```python
from build123d import *

# Parameters (mm, degrees)
F3_R        = 22.5
F4_DEPTH    = 80
F2_R        = 7.5
F0_R        = 17.5
F4_FACE_R   = 22.5
F4_FACE_R_2 = 7.5
F6_DEPTH    = 2


with BuildPart() as f4:
    # F3 (on Top) → F4 (new body)
    with BuildSketch(Plane.XY):
        Circle(F3_R)
    extrude(amount=F4_DEPTH)

    # F2 (on offset) → F5 section 0
    with BuildSketch(Plane.XY.offset(80)):
        Circle(F2_R)
    # F0 (on Top) → F5 section 1
    with BuildSketch(Plane.XY):
        Circle(F0_R)
    loft(mode=Mode.SUBTRACT)

    # F2 (on offset) + F4_face (on face) → F6 (join)
    with BuildSketch(Plane.XY.offset(80)):
        Circle(F2_R)
    with BuildSketch(Plane.XY.offset(80)):
        Circle(F4_FACE_R)
        Circle(F4_FACE_R_2, mode=Mode.SUBTRACT)
    extrude(amount=F6_DEPTH)


solid = f4.part
```
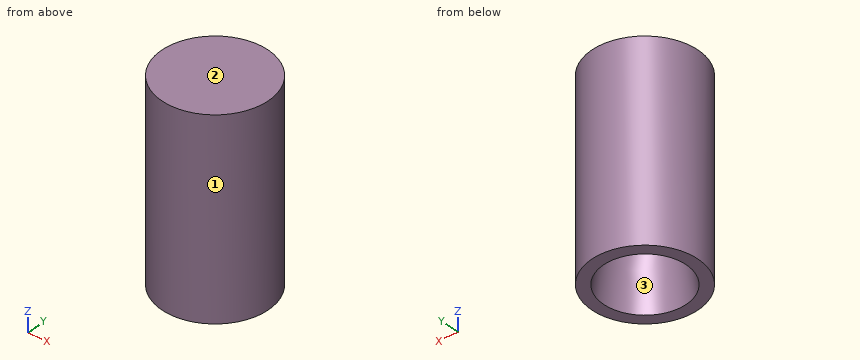
Model file for the job. Use its own axes, mm. Face numbers are marked on the shaded views. Give positions to 0.01 mm unless a question says otherwise; leave off trailing zeros. Order: outer loops, then holes, each group sorted by start corner. A loop starts at its lowest first (then second) coordinate and runs counter-clockwise, first axis right, second up.
1) Mould opens along X. For the marked faces 1, 2 and 3 say: +X half, -X half, draft (parallel to the pull), parting line (faces both ways), or undercut.
2) Saw through at C-C, the plane z = 74. Write the cut outline in (x, y), then the cut area to 3 significant figures.
3) Saw through at B-B, the plane z = 34. Write the cut outline in (x, y), then the cut area to 3 significant figures.
4) Saw through at A-A, the plane x = 0. Write the cut outline in (y, z), then the cut area to 3 significant figures.
5) Wall check: probe 1 along X at (y, z) = (-8.5, 57); probe 2 along Z at (x, y) = (-5.5, -3); probe 3 along X at (y, z) = (-5.5, 9.5). Give the ranges that are in metal, low to high.
6) Pin check, flat tips, straight feed: pin 1 (6 mm diameter, centred on x = 8, z = 40, fed in from +Y); pin 2 (1.5 mm diameter, centred on y = -16.5, z = 38, fed in from +X); pin 3 (1.5 mm diameter, centred on x = 1.5, z = 66, fed in from +Y); pin 4 (8 mm diameter, centred on y = -1, z = 24.5, fed in from -X). Stop position of each tip, or through.
Computed:
1. face 1: parting line
1. face 2: draft
1. face 3: undercut
2. outline: circle Ø45 at (0, 0); hole circle Ø16.5 at (0, 0)
2. area: 1,380 mm2
3. outline: circle Ø45 at (0, 0); hole circle Ø26.5 at (0, 0)
3. area: 1,040 mm2
4. outline: (-22.5, 0) - (-17.5, 0) - (-7.5, 80) - (7.5, 80) - (17.5, 0) - (22.5, 0) - (22.5, 82) - (-22.5, 82) - close
4. area: 1,690 mm2
5. probe 1: x = -20.83 to -5.95, 5.95 to 20.83
5. probe 2: z = 80 to 82
5. probe 3: x = -21.82 to -15.36, 15.36 to 21.82
6. pin 1: stops at y = 21.94
6. pin 2: stops at x = 16.07
6. pin 3: stops at y = 22.49
6. pin 4: stops at x = -22.5
